Autodesk Inventor part; units mm, degrees
ref_plane "YZ Plane" through (0, 0, 0) normal (1, 0, 0) x (0, 1, 0)
ref_plane "XZ Plane" through (0, 0, 0) normal (0, 1, 0) x (-1, 0, 0)
ref_plane "XY Plane" through (0, 0, 0) normal (0, 0, 1) x (1, 0, 0)
sketch "Sketch1" plane through (0, 0, 0) normal (0, 1, 0) x (-1, 0, 0)
  line L0 (50, 15) -> (-50, 15)
  line L1 (-50, 15) -> (-50, -15)
  line L2 (-50, -15) -> (50, -15)
  line L3 (50, -15) -> (50, 15)
  line L4 (50, 15) -> (-50, -15) construction
  line L5 (-50, 15) -> (50, -15) construction
  point P0 (0, 0)
  dimension "d0" = 100
  dimension "d1" = 30
extrude "Extrusion1" add sketch "Sketch1" along normal blind 3
sketch "Sketch2" plane through (50, 0, 15) normal (1, 0, 0) x (0, 0, -1)
  line L0 (0, 0) -> (3, 3)
  line L1 (0, 0) -> (4.2426, 0) construction
  line L2 (3, 3) -> (0, 3)
  line L3 (0, 0) -> (0, 3)
  line L4 (0, 3) -> (0, 0)
  dimension "d4" = 45
extrude "Extrusion2" cut sketch "Sketch2" against normal blind 100
sketch "Sketch3" plane through (0, 0, 0) normal (0, -1, 0) x (1, 0, 0)
  line L0 (25, -15) -> (-25, -15)
  line L1 (-25, -15) -> (-25, -3)
  line L2 (-25, -3) -> (25, -3)
  line L3 (25, -3) -> (25, -15)
  line L4 (0, 0) -> (0, -9.0285)
  line L5 (50, -15) -> (-50, -15)
  circle A0 centre (42, 0) radius 1.75
  circle A1 centre (-42, 0) radius 1.75
  line L6 (25, -3) -> (34, -15)
  line L7 (34, -15) -> (25, -15)
  line L8 (-25, -3) -> (-34, -15)
  line L9 (-25, -15) -> (-34, -15)
  line L10 (50, 15) -> (50, -15)
  dimension "d7" = 50
  dimension "d8" = 12
  dimension "d9" = 0
  dimension "d10" = 3.5
  dimension "d12" = 15
  dimension "d19" = 9
  dimension "d20" = 9
  dimension "d21" = 8
extrude "Extrusion3" cut sketch "Sketch3" against normal through all
chamfer "Chamfer1" distance 2 angle 45 2 edges at (40.25, 0, 0) (-43.75, 0, 0)
fillet "Fillet1" radius 2 4 edges at (-25, 1.5, -3) (25, 1.5, -3) (-34, 1.5, -15) (34, 1.5, -15)
properties part number "HM_Knife_cut" material "Steel, Alloy"
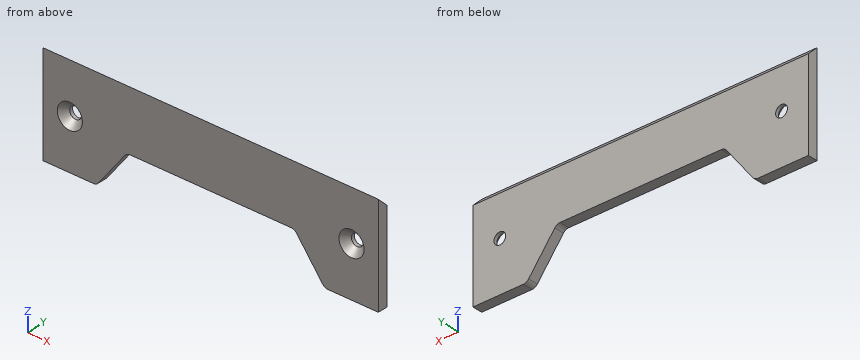
Verification items for the finished model (mm, model axes). Coordinates: 2 decimals unless noted, no trailing zeros. Write each loop counter-clockwise with the first axis right and the second up, starting at its lowest first coordinate (ties: lowest second). Pieces come first, ordered by that corner, then holes. Notation, with made-up numbers: M 17,-35.5 L 41,-35.5 A36 ccw 41,1.5 Z; hole C 54.25,49 d1. An arc over 180 degrees is marked long. Use a Markdown table: item, result.
Q1. Sectioned sample at C-C, the plane y = 1.3. Record the boundary of the cut face in (x, z), plus the area to 3 significant figures.
Reply:
| item | result |
|---|---|
| outline | M -50,-15 L -35,-15 A2 ccw -33.4,-14.2 L -25.6,-3.8 A2 cw -24,-3 L 24,-3 A2 cw 25.6,-3.8 L 33.4,-14.2 A2 ccw 35,-15 L 50,-15 L 50,13.7 L -50,13.7 Z; hole C -42,0 d4.9; hole C 42,0 d4.9 |
| area | 2,120 mm² |
Q2. Thickness scan on line 1 (Z direction, x = 42, y = 2.85); line 2 (Z direction, x = 40.5, y = 0.8); line 3 (X direction, y = 1.05, z = -7.75). Record the ranges inside material, lowest first.
Reply:
| item | result |
|---|---|
| line 1 | z = -15 to -1.75, 1.75 to 12.15 |
| line 2 | z = -15 to -2.54, 2.54 to 14.2 |
| line 3 | x = -50 to -28.56, 28.56 to 50 |
Q3. Sectioned sample at A-A, the plane x = -42. Record the boundary of the cut face in (y, z).
Reply:
| item | result |
|---|---|
| outline | M 0,-15 L 3,-15 L 3,-1.75 L 2,-1.75 L 0,-3.75 Z; M 0,3.75 L 2,1.75 L 3,1.75 L 3,12 L 0,15 Z |
Q4. Go/stop test with flat-tipped pins: P1, Ø1.5, axis at x = -11, y = 1, coming from the -Z side; P2, Ø2, axis at x = 42, z = 0, coming from the -Y side. Record where each tip stops, or that it passes through.
Reply:
| item | result |
|---|---|
| P1 | stops at z = -3 |
| P2 | passes through |
Q5. Sectioned sample at D-D, the plane z = -11. Record the boundary of the cut face in (x, y).
Reply:
| item | result |
|---|---|
| outline | M -50,0 L -31,0 L -31,3 L -50,3 Z; M 31,0 L 50,0 L 50,3 L 31,3 Z |
Q6. Sectioned sample at B-B, the plane z = 0. Record the boundary of the cut face in (x, y).
Reply:
| item | result |
|---|---|
| outline | M -50,0 L -45.75,0 L -43.75,2 L -43.75,3 L -50,3 Z; M -40.25,2 L -38.25,0 L 38.25,0 L 40.25,2 L 40.25,3 L -40.25,3 Z; M 43.75,2 L 45.75,0 L 50,0 L 50,3 L 43.75,3 Z |
